Study the drawing (mm; zero at the part's minimum x, y, z) and answer. Round coordinates to 2 decimals unless told otherwise and drop trailing zeros. Loops run counter-clockwise (first coordinate to the right, second up) from the corner with the lowest first, then second, coordinate; pieces in that order, holes last. Notation, with made-up numbers: (-9.75, -10) -> (-3.75, -10) arc R21 ccw to (-3.75, 5) -> close; hole circle Ø8 at (16, -34.75). An arc over 180 degrees is marked (long way). Write each question's results on one line, items separated by ' | '. Start each with the question number.
(1) Determine the mould class of the marked faces 1, 2, 3 and 4 for opening direction X: released by +X, released by -X, zero draft, split by the parting line, or undercut.
(2) The part is cut by section D-D (x = 87.5). Determine the outline of the cut face in (y, z), plus the area to 3 significant figures.
(3) Straight lines are drawn through the part: probe 1 along Z at (x, y) = (10, 41.5); probe 2 along X at (y, z) = (25, 94) (1 decimal); probe 3 along Z at (x, y) = (54, 23.5). For each, find the intervals that lie inside material, in ascending order.
(4) The part is cut by section C-C (y = 19.5). Determine the outline of the cut face in (x, z) (1 decimal).
(5) The part is cut by section A-A (z = 124.5). Determine the outline of the cut face in (x, y), plus the area to 3 significant figures.
(6) Flat-ended cylindrical pins translate along their axes: pin 1 (4 mm diameter, centred on y = 24, z = 122, fed in from +X) (1 decimal); pin 2 (6 mm diameter, centred on x = 52, y = 25.5, fed in from +Z); pin 3 (8 mm diameter, centred on x = 16.5, y = 5.5, fed in from +Z). Find the tip coordinate at first contact, or state that the pin passes through.
(7) The part is cut by section B-B (x = 72). Determine the outline of the cut face in (y, z) (1 decimal).
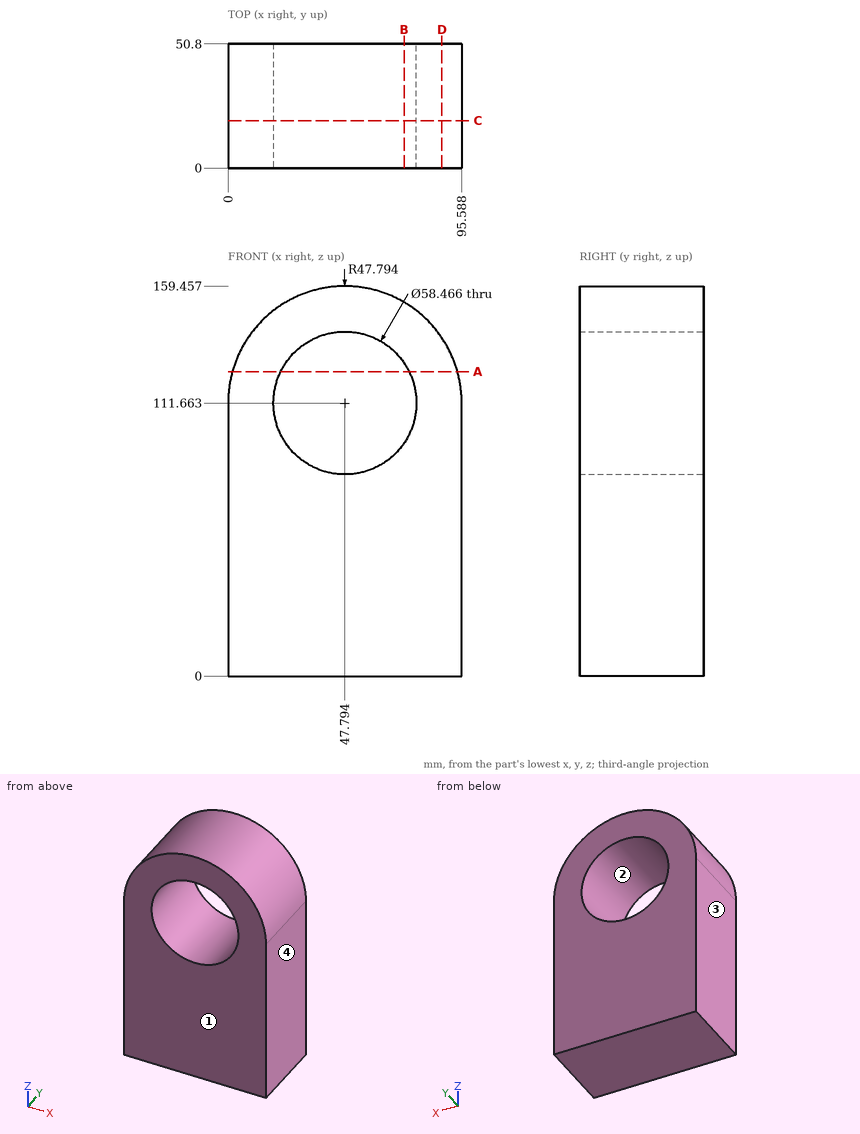
Checked values:
1) face 1: zero draft | face 2: undercut | face 3: released by -X | face 4: released by +X
2) outline: (0, 0) -> (50.8, 0) -> (50.8, 138.27) -> (0, 138.27) -> close | area: 7,020 mm2
3) probe 1: z = 0 to 140.92 | probe 2: x = 0 to 24.5, 71.1 to 95.6 | probe 3: z = 0 to 83.1, 140.23 to 159.05
4) outline: (0, 0) -> (95.6, 0) -> (95.6, 111.7) arc R47.8 ccw to (0, 111.7) -> close; hole circle Ø58.5 at (47.8, 111.7)
5) outline: (1.76, 0) -> (21.53, 0) -> (21.53, 50.8) -> (1.76, 50.8) -> close; (74.06, 0) -> (93.83, 0) -> (93.83, 50.8) -> (74.06, 50.8) -> close | area: 2,010 mm2
6) pin 1: stops at x = 94.9 | pin 2: stops at z = 159.44 | pin 3: stops at z = 150.9
7) outline: (0, 0) -> (50.8, 0) -> (50.8, 95.3) -> (0, 95.3) -> close; (0, 128.1) -> (50.8, 128.1) -> (50.8, 152.9) -> (0, 152.9) -> close
